```python
from build123d import *

# Parameters (mm, degrees)
ESQUISSE1_R             = 6.3
BOSS_EXTRU_1_DEPTH      = 5
ENL_V_MAT_EXTRU_1_DEPTH = 5
ESQUISSE3_W             = 5
ESQUISSE3_H             = 15
BOSS_EXTRU_3_DEPTH      = 5


with BuildPart() as part:
    # Esquisse1 → Boss.-Extru.1 (new body)
    with BuildSketch(Plane.XY):
        Polygon((-65, 51.461253746), (0, 40), (0, -40), (-9.359100785, -41.650261983), (-6.809077296, -56.112163836), (-31.918247866, -60.539588071), (-29.710027076, -73.063030491), (25, -63.416176602), (25, 63.800831685), (-18.444412366, 71.461253746), (-65, 71.461253746), align=None)
        with Locations((-20, 53.680805733)):
            Circle(ESQUISSE1_R, mode=Mode.SUBTRACT)
        with Locations(Location((10, -5, 0), (0, 0, 180))):
            Circle(ESQUISSE1_R, mode=Mode.SUBTRACT)
    extrude(amount=BOSS_EXTRU_1_DEPTH)

    # Esquisse2 → Enlèv. mat.-Extru.1 (cut)
    with BuildSketch(Plane(origin=(0, 0, 0), x_dir=(-1, 0, 0), z_dir=(0, 0, -1))):
        Polygon((31.396602506, -63.497985917), (30.230971609, -70.108607232), (25.306932844, -69.240366344), (26.472563741, -62.629745029), align=None)
    extrude(amount=-ENL_V_MAT_EXTRU_1_DEPTH, mode=Mode.SUBTRACT)

    # Esquisse3 → Boss.-Extru.3 (add)
    with BuildSketch(Plane.XY):
        Polygon((0, -40), (0, -30), (-5, -30), (-5, -35.804501844), (-0.868240888, -35.075961235), align=None)
        with Locations((-2.5, -5)):
            Rectangle(ESQUISSE3_W, ESQUISSE3_H)
        Polygon((-0.868240888, 35.075961235), (0, 40), (0, 25), (-5, 25), (-5, 35.804501844), align=None)
        Polygon((-29.122539924, 45.135089535), (-14.350423629, 42.53036687), (-15.218664517, 37.606328105), (-29.990780813, 40.21105077), align=None)
        Polygon((-65, 51.461253746), (-65, 46.384120687), (-55.15192247, 44.64763891), (-54.283681582, 49.571677675), align=None)
    extrude(amount=BOSS_EXTRU_3_DEPTH)


solid = part.part
```
Source: CAD feature listing. Evaluate the final solid. Frame: model axes, mm. A direction names the side the tool comes from. Give positions to 0.01 mm unless a question says otherwise; leave off trailing zeros. Write each loop counter-clockwise with the first axis right and the second up, starting at its lowest first coordinate (ties: lowest second). Pieces come first, ordered by that corner, then holes.
1. First-contact query: pin 1 (1.5 mm diameter, centred on y = -4.5, z = 2.5, fed in from -X); pin 2 (1 mm diameter, centred on x = -0.5, z = 1, fed in from -Y); pin 3 (2.5 mm diameter, centred on x = -3.5, z = 2.5, fed in from +Y); pin 4 (10 mm diameter, centred on x = -20, y = 53.68, fed in from -Z). Flat tips, straight axial feed; report the tip coordinate or a pass-through.
2. Section query C-C (x = 10). Return the cut outline in (y, z), then the cut area to 3 significant figures.
3. Material intervals for line 1 along Y through (x, z) = (-20, 3.2); line 2 along Y through (x, z) = (-27, 4.35); line 3 along Y through (x, z) = (10, 2.75), sorted ascending.
4. Section query B-B (x = -20). Return the cut outline in (y, z), then the cut area to 3 significant figures.
5. Pull-direction query (X, two-part tool) for faces 6 (the face through (-41, 71.461, 2)), 7 (the face through (-28.9, -63.058, 2.465)), 8 (the face through (-2.963, 35.445, 2.465)), 9 (the face through (-19.188, -58.295, 2.465)); classes: +X half, -X half, draft (parallel to the pull), parting line (faces both ways), or undercut.
6. Section query A-A (y = -5). Return the cut outline in (x, z).
7. Access query for faces 1 (the face through (-8.1, -48.8, 2.5)), 2 (the face through (-29.974, -71.565, 2.465)), 3 (the face through (-65, 59, 2)), 4 (the face through (-14.78, 40.1, 2.46)), 5 (the face through (-54.724, 47.075, 2.465)). Directions: +Z, -Z, +X, -X, +Y, -Y. A direction counts if a zero-diameter tool reaches every point of the face in a straight line with its end or side. Return the directions, or none.
8. Section query D-D (y = 31.5). Return the cut outline in (x, z).
Output values:
1. pin 1: stops at x = -5
1. pin 2: stops at y = -68
1. pin 3: stops at y = 69.05
1. pin 4: passes through
2. outline: (-66.06, 0) - (-11.3, 0) - (-11.3, 5) - (-66.06, 5) - close; (1.3, 0) - (66.45, 0) - (66.45, 5) - (1.3, 5) - close
2. area: 600 mm2
3. line 1: y = -71.35 to -58.44, 38.45 to 47.38, 59.98 to 71.46
3. line 2: y = -72.59 to -69.54, -62.72 to -59.67, 39.68 to 71.46
3. line 3: y = -66.06 to -11.3, 1.3 to 66.45
4. outline: (-71.35, 0) - (-58.44, 0) - (-58.44, 5) - (-71.35, 5) - close; (38.45, 0) - (47.38, 0) - (47.38, 5) - (38.45, 5) - close; (59.98, 0) - (71.46, 0) - (71.46, 5) - (59.98, 5) - close
4. area: 167 mm2
5. face 6: draft
5. face 7: undercut
5. face 8: undercut
5. face 9: -X half
6. outline: (-5, 0) - (3.7, 0) - (3.7, 5) - (-5, 5) - close; (16.3, 0) - (25, 0) - (25, 5) - (16.3, 5) - close
7. face 1: +Z, -Z, -X
7. face 2: +Z, -Z, -X, -Y
7. face 3: +Z, -Z, -X, +Y, -Y
7. face 4: +Z, -Z
7. face 5: +Z, -Z, -Y
8. outline: (-5, 0) - (25, 0) - (25, 5) - (-5, 5) - close
